Can you work these out from the drawing? Everything is in mm from the part's minimum corner. Give positions to 0.01 mm unless a question says otherwise; leave off trailing zeros. Order: outer loops, then holes, each group sorted by start corner. A loop starts at its lowest first (then second) coordinate and runs counter-clockwise, first axis right, second up. Notation, with made-up numbers: (6, -24) - (57, -24) arc R10 ccw to (57, -12) - close; hole circle Ø6 at (-20.75, 85.25). An arc over 180 degrees is marked (long way). One line per question, with ' | ' between items.
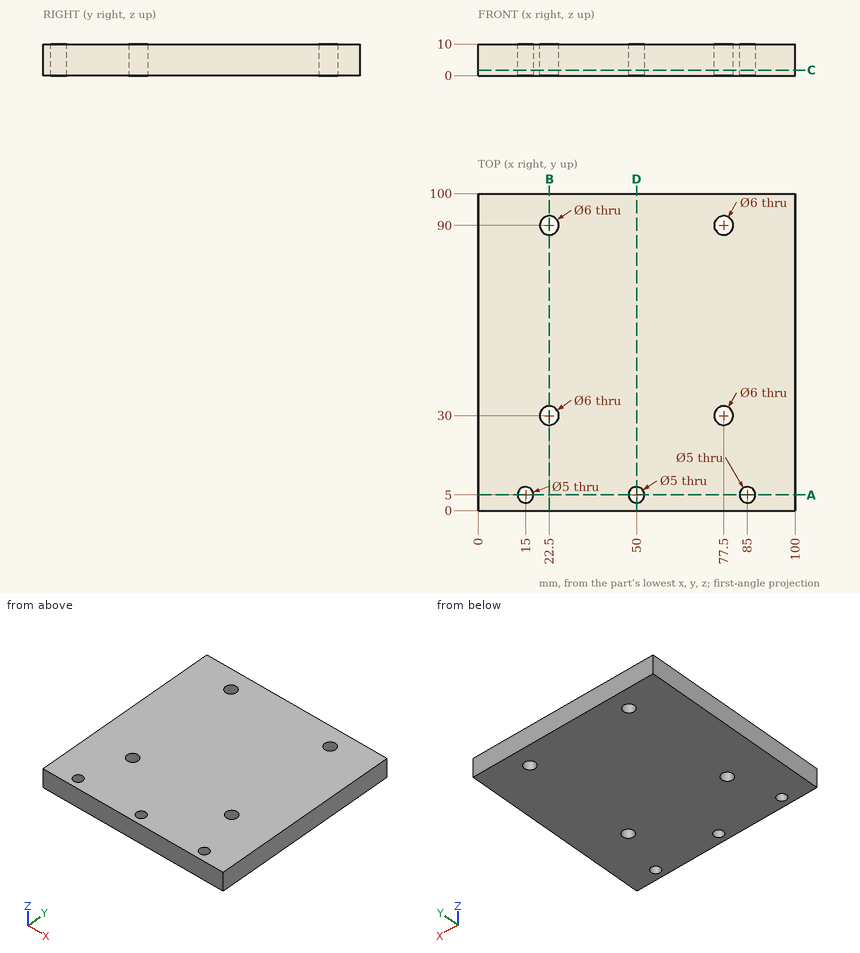
1) I'm going to push a flat-ended pin straight in: P1, Ø4, axis at x = 15, y = 5, coming from the -Z side. Where does the tip first touch, or does it pass through?
Model answer:
P1: passes through
2) I want a section at A-A (y = 5). List the corners of the cut face in (x, z) for me.
Model answer:
outline: (0, 0) - (12.5, 0) - (12.5, 10) - (0, 10) - close; (17.5, 0) - (47.5, 0) - (47.5, 10) - (17.5, 10) - close; (52.5, 0) - (82.5, 0) - (82.5, 10) - (52.5, 10) - close; (87.5, 0) - (100, 0) - (100, 10) - (87.5, 10) - close
3) I want a section at C-C (z = 1.75). List the corners of the cut face in (x, y) for me.
Model answer:
outline: (0, 0) - (100, 0) - (100, 100) - (0, 100) - close; hole circle Ø5 at (15, 5); hole circle Ø6 at (22.5, 30); hole circle Ø6 at (22.5, 90); hole circle Ø5 at (50, 5); hole circle Ø6 at (77.5, 30); hole circle Ø6 at (77.5, 90); hole circle Ø5 at (85, 5)
4) Please list where these lines run through material, in increasing order: L1, parallel to X at y = 30, z = 6.25; L2, parallel to Y at x = 15, z = 5.25; L3, parallel to Y at x = 77.5, z = 3.25.
Model answer:
L1: x = 0 to 19.5, 25.5 to 74.5, 80.5 to 100 | L2: y = 0 to 2.5, 7.5 to 100 | L3: y = 0 to 27, 33 to 87, 93 to 100
5) I want a section at D-D (x = 50). List the corners of the cut face in (y, z) for me, plus the area to 3 significant figures.
Model answer:
outline: (0, 0) - (2.5, 0) - (2.5, 10) - (0, 10) - close; (7.5, 0) - (100, 0) - (100, 10) - (7.5, 10) - close | area: 950 mm2
6) I want a section at B-B (x = 22.5). List the corners of the cut face in (y, z) for me, plus the area to 3 significant figures.
Model answer:
outline: (0, 0) - (27, 0) - (27, 10) - (0, 10) - close; (33, 0) - (87, 0) - (87, 10) - (33, 10) - close; (93, 0) - (100, 0) - (100, 10) - (93, 10) - close | area: 880 mm2
